Verification items for this drawing (mm, ordinates from the low corner). Round coordinates to 2 decimals unless told otherwise and drop trailing zeros. Write each loop counter-clockwise with the first axis right and the second up, starting at its lowest first coordinate (ties: lowest second). Pieces come first, ordered by that corner, then holes.
Item 1: Cross-section at A-A (y = 21.36). Enter the section's corners in (x, z), then the cut area to 3 significant figures.
Item 2: Cross-section at B-B (x = 12.53). Enter the section's corners in (y, z), then the cut area to 4 significant figures.
Item 3: Cross-section at C-C (z = 0.8). Enter the section's corners in (x, y), then the cut area to 3 significant figures.
Item 4: Scan lines: probe 1 along Y at (x, z) = (1.25, 0.2); probe 2 along Y at (x, z) = (12.53, 0.5); probe 3 along Y at (x, z) = (11, 0.65). Record each from-to range of solid material in increasing order.
Item 5: Depth check by flat-ended pin: P1, Ø0.5, axis at y = 18, z = 0.5, coming from the +X side. Enter the tip coordinate at first touch or a pass-through.
Item 6: Cross-section at D-D (x = 1.5). Enter the section's corners in (y, z).
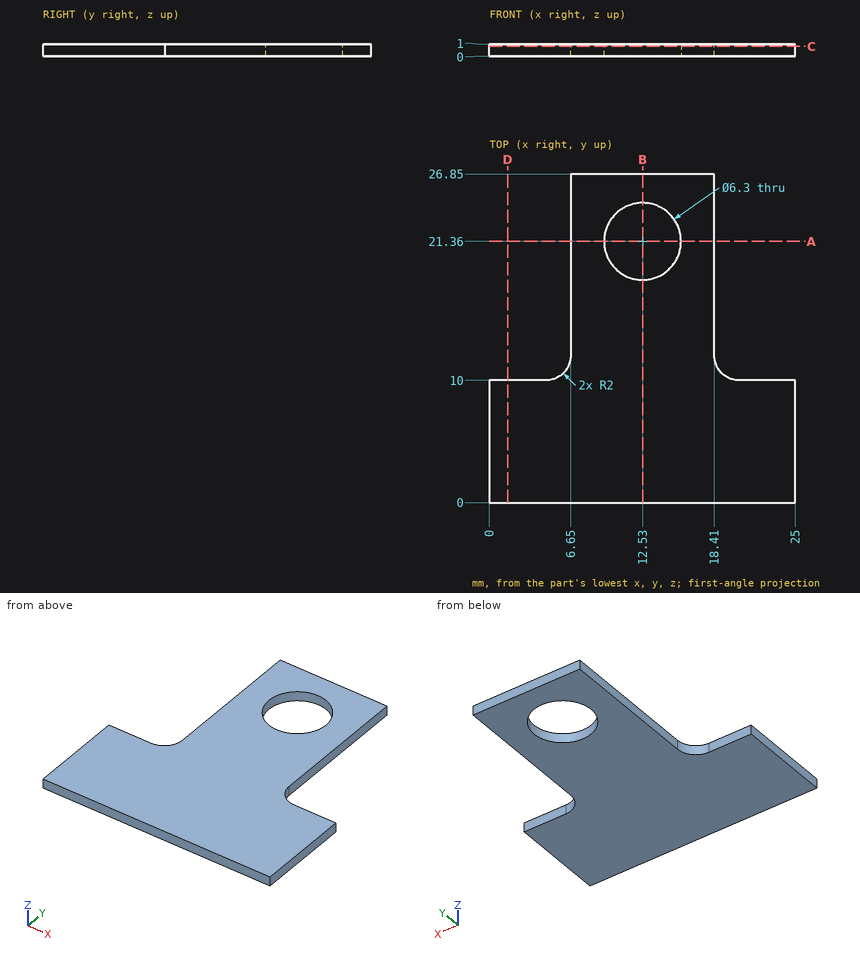
Resolved:
1. outline: (6.65, 0) - (9.38, 0) - (9.38, 1) - (6.65, 1) - close; (15.68, 0) - (18.41, 0) - (18.41, 1) - (15.68, 1) - close
1. area: 5.46 mm2
2. outline: (0, 0) - (18.21, 0) - (18.21, 1) - (0, 1) - close; (24.51, 0) - (26.85, 0) - (26.85, 1) - (24.51, 1) - close
2. area: 20.55 mm2
3. outline: (0, 0) - (25, 0) - (25, 10) - (20.41, 10) arc R2 cw to (18.41, 12) - (18.41, 26.85) - (6.65, 26.85) - (6.65, 12) arc R2 cw to (4.65, 10) - (0, 10) - close; hole circle Ø6.3 at (12.53, 21.36)
3. area: 419 mm2
4. probe 1: y = 0 to 10
4. probe 2: y = 0 to 18.21, 24.51 to 26.85
4. probe 3: y = 0 to 18.61, 24.11 to 26.85
5. P1: stops at x = 18.41
6. outline: (0, 0) - (10, 0) - (10, 1) - (0, 1) - close
